from build123d import *

# Parameters (mm, degrees)
SKETCH1_R               = 3.175
BOSS_EXTRUDE1_DEPTH     = 3.175
SKETCH2_W               = 63.5
SKETCH2_H               = 3.175
BOSS_EXTRUDE2_DEPTH     = 25.4
CUT_EXTRUDE1_DEPTH      = 105.410975214
CUT_EXTRUDE1_DEPTH_BACK = 105.410975214
SKETCH3_R               = 3.175


with BuildPart() as part:
    # Sketch1 → Boss-Extrude1 (new body)
    with BuildSketch(Plane.XY):
        with BuildLine():
            Line((0, 78.705067014), (0, 0))
            Line((0, 0), (63.5, 0))
            Line((63.5, 0), (63.5, 15.875))
            Line((63.5, 15.875), (15.080341671, 64.294658329))
            ThreePointArc((15.080341671, 64.294658329), (8.505408108, 64.65221549), (11.339511683, 70.595737627))
            ThreePointArc((11.339511683, 70.595737627), (12.906539417, 71.462906002), (13.511840983, 73.148482141))
            ThreePointArc((13.511840983, 73.148482141), (8.586326617, 80.377738088), (0, 78.705067014))
        make_face()
        with Locations((9.525, 22.225)):
            Circle(SKETCH1_R, mode=Mode.SUBTRACT)
        with Locations((41.275, 22.225)):
            Circle(SKETCH1_R, mode=Mode.SUBTRACT)
        with Locations((9.525, 53.975)):
            Circle(SKETCH1_R, mode=Mode.SUBTRACT)
    extrude(amount=BOSS_EXTRUDE1_DEPTH)

    # Sketch2 → Boss-Extrude2 (add)
    with BuildSketch(Plane.XY.offset(3.175)):
        with Locations((31.75, 1.5875)):
            Rectangle(SKETCH2_W, SKETCH2_H)
    extrude(amount=BOSS_EXTRUDE2_DEPTH)

    # Sketch3 → Cut-Extrude1 (cut, two sides: drawn at the far end of the back side and taken through both)
    with BuildSketch(Plane(origin=(0, 3.175, 0), x_dir=(1, 0, 0), z_dir=(0, 1, 0)).offset(-CUT_EXTRUDE1_DEPTH_BACK)):
        with Locations(Location((9.525, -19.05, 0), (0, 0, 270))):
            Circle(SKETCH3_R)
        with Locations(Location((53.975, -19.05, 0), (0, 0, 270))):
            Circle(SKETCH3_R)
        with Locations(Location((31.75, -15.875, 0), (0, 0, 270))):
            Circle(SKETCH3_R)
    extrude(amount=CUT_EXTRUDE1_DEPTH + CUT_EXTRUDE1_DEPTH_BACK, mode=Mode.SUBTRACT)


solid = part.part
Here's how the part is built. I have some questions about the finished solid (model axes, mm). A direction names the side the tool comes from. Coordinates: 2 decimals unless noted, no trailing zeros. Order: outer loops, then holes, each group sorted by start corner. A loop starts at its lowest first (then second) coordinate and runs counter-clockwise, first axis right, second up. Notation, with made-up numbers: (7.25, 10) -> (19.25, 10) arc R13 cw to (19.25, 15) -> close; hole circle Ø11 at (15.25, 68). An arc over 180 degrees is marked (long way). Answer in a Markdown table with one row per item.
(1) On a 3-axis mill with a long thin cutter (end or side, diameter ignored), from which of +Z, -Z, +X, -X, +Y, -Y can I reach the whole of each face in a straight line? I mean faces 1 (the face through (12.89, 71.443, 1.565)), 2 (the face through (31, 3.175, 10)), 3 (the face through (9.665, 1.565, 15.878)). Say none if no direction works.
Answer key:
| item | result |
|---|---|
| face 1 | +Z, -Z, +X |
| face 2 | +Z, +X, -X, +Y |
| face 3 | +Y, -Y |
(2) I want a section at B-B on z = 20.25. List the corners of the cut face in (x, y) for me (1 decimal), then the cut area to 3 significant figures.
Answer key:
| item | result |
|---|---|
| outline | (0, 0) -> (6.6, 0) -> (6.6, 3.2) -> (0, 3.2) -> close; (12.5, 0) -> (51, 0) -> (51, 3.2) -> (12.5, 3.2) -> close; (56.9, 0) -> (63.5, 0) -> (63.5, 3.2) -> (56.9, 3.2) -> close |
| area | 164 mm^2 |
(3) I want a section at A-A on x = 31.75. List the corners of the cut face in (y, z) for me (3 decimals), then the cut area to 3 significant figures.
Answer key:
| item | result |
|---|---|
| outline | (0, 0) -> (47.625, 0) -> (47.625, 3.175) -> (3.175, 3.175) -> (3.175, 12.7) -> (0, 12.7) -> close; (0, 19.05) -> (3.175, 19.05) -> (3.175, 28.575) -> (0, 28.575) -> close |
| area | 212 mm^2 |
(4) Please list where these lines run through material, in increasing order: probe 1 along Z at (x, y) = (37, 38) (3 decimals); probe 2 along X at (y, z) = (69, 1.75).
Answer key:
| item | result |
|---|---|
| probe 1 | 0 to 3.175 |
| probe 2 | 0 to 8.7 |
(5) I want a section at D-D on z = 9.25. List the corners of the cut face in (x, y) for me (3 decimals), then the cut area to 3 significant figures.
Answer key:
| item | result |
|---|---|
| outline | (0, 0) -> (63.5, 0) -> (63.5, 3.175) -> (0, 3.175) -> close |
| area | 202 mm^2 |
(6) I want a section at C-C on y = 32. List the corners of the cut face in (x, z) for me (3 decimals), then the cut area to 3 significant figures.
Answer key:
| item | result |
|---|---|
| outline | (0, 0) -> (47.375, 0) -> (47.375, 3.175) -> (0, 3.175) -> close |
| area | 150 mm^2 |
(7) Will these pins go through, and if not, where does the flat tip stop? pin 1 Ø6.5 at (x, y) = (11.91, 66.67) entering from -Z; pin 2 Ø12.5 at (x, z) = (38, 13) entering from +Y (3 decimals); pin 3 Ø7.5 at (x, y) = (41.275, 22.225) entering from +Z (3 decimals).
Answer key:
| item | result |
|---|---|
| pin 1 | through |
| pin 2 | y = 3.175 |
| pin 3 | z = 3.175 |
(8) Thinking about a two-plate mould opening in Z: for faces 4 (the face through (24, 32, 0)), 5 (the face through (52.043, 1.565, 16.53)), 6 (the face through (0, 30, 3)), which applies, +Z half, -Z half, draft (parallel to the pull), parting line (faces both ways), or undercut?
Answer key:
| item | result |
|---|---|
| face 4 | -Z half |
| face 5 | undercut |
| face 6 | draft |
